Check sheet for the drawn part. Datum: minimum x, y, z corner. Units: mm. Give positions to 0.01 mm unless a question says otherwise; leave off trailing zeros. Write each loop counter-clockwise with the first axis right and the second up, starting at its lowest first coordinate (ties: lowest second). Pieces come first, ordered by that corner, then holes.
(1) Cross-section at C-C (x = 73). Record the boundary of the cut face in (y, z).
(2) Cross-section at A-A (y = 33). Record the boundary of the cut face in (x, z).
(3) Cross-section at B-B (z = 3.1). Record the boundary of the cut face in (x, y).
(4) Mould release check, pull along Y, two halves, no side actions. Record for the marked faces 1 and 2: +Y half, -Y half, draft (parallel to the pull), parting line (faces both ways), or undercut.
(5) Thickness scan on line 1 along X through (y, z) = (44.5, 1.95); line 2 along Y through (x, z) = (78, 3.05); line 3 along X through (y, z) = (31, 2.1). Record the ranges inside material, lowest first.
(6) Cross-section at D-D (y = 21). Record the boundary of the cut face in (x, z), and give its area (3 significant figures).
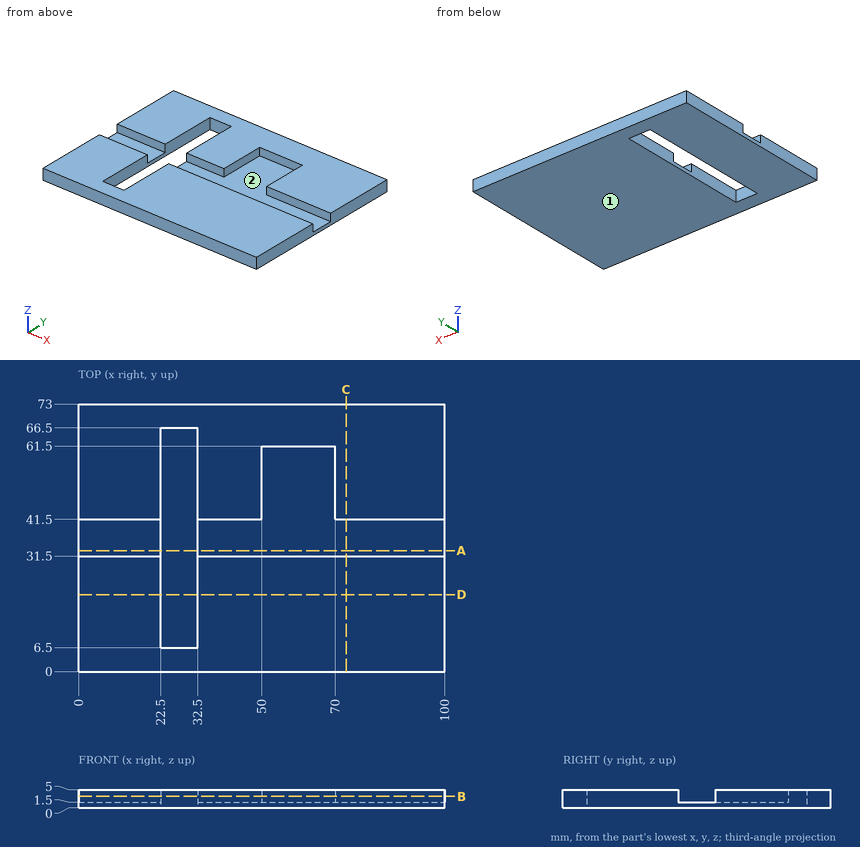
Reply:
1. outline: (0, 0) - (73, 0) - (73, 5) - (41.5, 5) - (41.5, 1.5) - (31.5, 1.5) - (31.5, 5) - (0, 5) - close
2. outline: (0, 0) - (22.5, 0) - (22.5, 1.5) - (0, 1.5) - close; (32.5, 0) - (100, 0) - (100, 1.5) - (32.5, 1.5) - close
3. outline: (0, 0) - (100, 0) - (100, 31.5) - (32.5, 31.5) - (32.5, 6.5) - (22.5, 6.5) - (22.5, 31.5) - (0, 31.5) - close; (0, 41.5) - (22.5, 41.5) - (22.5, 66.5) - (32.5, 66.5) - (32.5, 41.5) - (50, 41.5) - (50, 61.5) - (70, 61.5) - (70, 41.5) - (100, 41.5) - (100, 73) - (0, 73) - close
4. face 1: draft
4. face 2: undercut
5. line 1: x = 0 to 22.5, 32.5 to 50, 70 to 100
5. line 2: y = 0 to 31.5, 41.5 to 73
5. line 3: x = 0 to 22.5, 32.5 to 100
6. outline: (0, 0) - (22.5, 0) - (22.5, 5) - (0, 5) - close; (32.5, 0) - (100, 0) - (100, 5) - (32.5, 5) - close
6. area: 450 mm2
